from build123d import *

# Parameters (mm, degrees)
PAD_DEPTH       = 4
SKETCH001_R     = 2
SKETCH001_W     = 0.85
SKETCH001_H     = 2.6
POCKET_DEPTH    = 10
SKETCH002_W     = 11.8
SKETCH002_H     = 3.6
POCKET001_DEPTH = 15
SKETCH003_W     = 11.8
SKETCH003_H     = 0.8
POCKET002_DEPTH = 5


with BuildPart() as part:
    # Sketch → Pad (new body, symmetric)
    with BuildSketch(Plane.YZ):
        with BuildLine():
            Line((-5.45, -14.8), (-5.45, -0.5))
            ThreePointArc((-4.95, 0), (-5.303553, -0.146447), (-5.45, -0.5))
            Line((-4.95, 0), (4.95, 0))
            ThreePointArc((5.45, -0.5), (5.303553, -0.146447), (4.95, 0))
            Line((5.45, -0.5), (5.45, -14.8))
            Line((5.45, -14.8), (4.65, -14.8))
            Line((4.65, -14.8), (4.65, -0.8))
            Line((4.65, -0.8), (-4.65, -0.8))
            Line((-4.65, -0.8), (-4.65, -14.8))
            Line((-4.65, -14.8), (-5.45, -14.8))
        make_face()
    extrude(amount=PAD_DEPTH, both=True)

    # Sketch001 (on Face9 of Pad) → Pocket (cut)
    with BuildSketch(Plane(origin=(0, 0, 0), x_dir=(0, -1, 0), z_dir=(0, 0, 1))):
        Circle(SKETCH001_R)
        with Locations((-5.025, 2.7)):
            Rectangle(SKETCH001_W, SKETCH001_H)
        with Locations((-5.025, -2.7)):
            Rectangle(SKETCH001_W, SKETCH001_H)
        with Locations((5.025, 2.7)):
            Rectangle(SKETCH001_W, SKETCH001_H)
        with Locations((5.025, -2.7)):
            Rectangle(SKETCH001_W, SKETCH001_H)
    extrude(amount=-POCKET_DEPTH, mode=Mode.SUBTRACT)

    # Sketch002 (on Face24 of Pocket) → Pocket001 (cut)
    with BuildSketch(Plane(origin=(0, -5.45, 0), x_dir=(0, 0, -1), z_dir=(0, -1, 0))):
        with Locations((8.9, 2.2)):
            Rectangle(SKETCH002_W, SKETCH002_H)
        with Locations((8.9, -2.2)):
            Rectangle(SKETCH002_W, SKETCH002_H)
    extrude(amount=-POCKET001_DEPTH, mode=Mode.SUBTRACT)

    # Sketch003 (on Face24 of Pocket001) → Pocket002 (cut)
    with BuildSketch(Plane(origin=(0, -5.45, 0), x_dir=(0, 0, -1), z_dir=(0, -1, 0))):
        with Locations((8.9, 0)):
            Rectangle(SKETCH003_W, SKETCH003_H)
    extrude(amount=-POCKET002_DEPTH, mode=Mode.SUBTRACT)


solid = part.part
Model file for the job. Use its own axes, mm. A direction names the side the tool comes from. Give positions to 0.01 mm unless a question says otherwise; leave off trailing zeros. Order: outer loops, then holes, each group sorted by start corner. A loop starts at its lowest first (then second) coordinate and runs counter-clockwise, first axis right, second up. Notation, with made-up numbers: (27.25, 29) - (65.25, 29) arc R14 ccw to (65.25, 35) - close; hole circle Ø7 at (64, -35.5). An arc over 180 degrees is marked (long way). Write item = value, one per line. Start each with the question number.
1. Cut at C-C, the plane x = 0. List the corners of the cut face in (y, z).
2. Cut at B-B, the plane z = -2.25. List the corners of the cut face in (x, y), and give its area (3 significant figures).
3. Cut at A-A, the plane y = 0. List the corners of the cut face in (x, z).
4. Which spindle directions (+Z, -Z, +X, -X, +Y, -Y) get a long thin tool onto all of the face, cutting with end or side? Do faces 1 (the flat face through (2, -1, 0)), 2 (the flat face through (-1.4, -5, -1)), 3 (the flat face through (2, 1, -0.8)), 4 (the flat face through (1.4, -5, -1)). Say none if no direction does.
5. Cut at D-D, the plane x = 3.5. List the corners of the cut face in (y, z).
6. Drop flat-ended pins along their axis: P1, Ø0.6, axis at y = 5, z = -7, coming from the -X side; P2, Ø4.5, axis at x = 0, y = 0, coming from the -Z side; P3, Ø0.9, axis at y = -5, z = -1.5, coming from the -X side. Give the stop position or say it passes through.
7. Two-plate mould, pull along X, no slides. Class faces 5 (the flat face through (-1.4, 5, -1)), 6 (the flat face through (1.4, 5, -1)), 7 (the flat face through (0, -4.65, -2)), 8 (the cylindrical face through (-1.952, 0.434, -0.394)): pulls with the +X half, pulls with the -X half, needs draft (parallel to the pull), parting line crosses it, or undercut.
8. Probe line 1 along Y through (x, z) = (-1.25, -2.25); line 2 along X through (y, z) = (0, -0.4); line 3 along Z through (x, y) = (-1.5, 3). List the from-to ranges inside material, lowest first.
Taken from the geometry:
q1.outline = (-5.45, -3) - (-4.65, -3) - (-4.65, -0.8) - (-2, -0.8) - (-2, 0) - (-4.95, 0) arc R0.5 ccw to (-5.45, -0.5) - close; (2, -0.8) - (4.65, -0.8) - (4.65, -14.8) - (5.45, -14.8) - (5.45, -0.5) arc R0.5 ccw to (4.95, 0) - (2, 0) - close
q2.outline = (-1.4, -5.45) - (1.4, -5.45) - (1.4, -4.65) - (-1.4, -4.65) - close; (-1.4, 4.65) - (1.4, 4.65) - (1.4, 5.45) - (-1.4, 5.45) - close
q2.area = 4.48 mm²
q3.outline = (-4, -0.8) - (-2, -0.8) - (-2, 0) - (-4, 0) - close; (2, -0.8) - (4, -0.8) - (4, 0) - (2, 0) - close
q4.face_1 = +Z, +X, -X, +Y, -Y
q4.face_2 = +Z, -Z, -X, -Y
q4.face_3 = -Z, +X, -X
q4.face_4 = +Z, -Z, +X, -Y
q5.outline = (-4.6, -0.8) - (4.6, -0.8) - (4.6, 0) - (-4.6, 0) - close
q6.P1 = -0.4
q6.P2 = -0.8
q6.P3 = -1.4
q7.face_5 = pulls with the -X half
q7.face_6 = pulls with the +X half
q7.face_7 = needs draft
q7.face_8 = undercut
q8.line_1 = -5.45 to -4.65, 4.65 to 5.45
q8.line_2 = -4 to -2, 2 to 4
q8.line_3 = -0.8 to 0
